Input: part model. Units: mm. Frame: model coordinates. A direction names the side the tool comes from. Give positions to 0.01 mm unless a question says otherwise; leave off trailing zeros. Loops run counter-clockwise (first coordinate to the right, second up) from the corner with the lowest first, then second, coordinate; pieces in that order, holes last.
from build123d import *

# Parameters (mm, degrees)
SKETCH1_R           = 5.375
SKETCH1_R_2         = 3.375
BOSS_EXTRUDE1_DEPTH = 12
FILLET1_R           = 10
FILLET1_2_R         = 6
CHAMFER1_SIZE       = 1


with BuildPart() as part:
    # Sketch1 → Boss-Extrude1 (new body)
    with BuildSketch(Plane.XY):
        Circle(SKETCH1_R)
        Circle(SKETCH1_R_2, mode=Mode.SUBTRACT)
        with BuildLine():
            Line((13.516056888, 82), (2.713546265, 82))
            Line((2.713546265, 82), (-5.348872315, 0.529329726))
            ThreePointArc((-5.348872315, 0.529329726), (0.264987082, 5.368464105), (5.375, 0))
            ThreePointArc((5.375, 0), (5.368464105, -0.264987082), (5.348872315, -0.529329726))
            Line((5.348872315, -0.529329726), (13.516056888, 82))
        make_face()
        Polygon((14.307744846, 90), (3.505234224, 90), (2.713546265, 82), (13.516056888, 82), align=None)
        Polygon((46.473934517, 90), (14.307744846, 90), (13.516056888, 82), (46.473934517, 82), align=None)
    extrude(amount=BOSS_EXTRUDE1_DEPTH)

    # Fillet1
    fillet1_edges = [part.edges().sort_by_distance(p)[0] for p in [
        (3.505234224, 90, 6),
    ]]
    fillet(fillet1_edges, radius=FILLET1_R)

    # Fillet1 2
    fillet1_2_edges = [part.edges().sort_by_distance(p)[0] for p in [
        (13.516056888, 82, 6),
    ]]
    fillet(fillet1_2_edges, radius=FILLET1_2_R)

    # Chamfer1
    chamfer1_edges = [part.edges().sort_by_distance(p)[0] for p in [
        (-0.529329726, -5.348872315, 12),
        (-0.529329726, -5.348872315, 0),
        (32.712766845, 82, 12),
        (9.164818638, 38.030774984, 0),
        (9.164818638, 38.030774984, 12),
        (-1.367895651, 40.757064607, 0),
        (-1.367895651, 40.757064607, 12),
        (29.519202941, 90, 0),
        (5.850604928, 87.411072625, 0),
        (29.519202941, 90, 12),
        (5.850604928, 87.411072625, 12),
        (14.92327931, 80.446643575, 0),
        (14.92327931, 80.446643575, 12),
        (32.712766845, 82, 0),
    ]]
    chamfer(chamfer1_edges, length=CHAMFER1_SIZE)


solid = part.part
(1) Mould query, pull axis Z, two halves, no side actions, for faces 1 (the cylindrical face through (-0.647, -5.336, 5.93)), 2 (the flat face through (8.607, 37.541, 11.507)), 3 (the flat face through (-0.822, 41.272, 0.507)). Classes: +Z half, -Z half, draft (parallel to the pull), parting line (faces both ways), or undercut.
Values follow:
face 1: draft
face 2: +Z half
face 3: -Z half
(2) Cut plane A-A (x = 29.5). Return the cut outline in (y, z).
Values follow:
outline: (82, 1) - (83, 0) - (89, 0) - (90, 1) - (90, 11) - (89, 12) - (83, 12) - (82, 11) - close
(3) Reachability of faces 4 (the flat face through (33, 82, 6)), 5 (the conical face through (14.76, 80.53, 11.17)) from +Z, -Z, +X, -X, +Y, -Y: full face, straight path, thin tool, end or side. Return the list, or none.
Values follow:
face 4: +Z, -Z, +X, -Y
face 5: +Z, +X, -Y
(4) Cut plane B-B (y = 2). Return the cut outline in (x, z), and give its area (3 significant figures).
Values follow:
outline: (-5.2, 1) - (-4.2, 0) - (-2.72, 0) - (-2.72, 12) - (-4.2, 12) - (-5.2, 11) - close; (2.72, 0) - (4.59, 0) - (5.6, 1) - (5.6, 11) - (4.59, 12) - (2.72, 12) - close
area: 62.4 mm2
(5) Pin query (flat end, axial travel): pin 1 Ø1 at (y, z) = (17, 7) entering from -X. Return the tip coordinate at first contact, or that it passes through.
Values follow:
pin 1: stops at x = -3.77
(6) Cut plane C-C (x = 0). Return the cut outline in (y, z) (3 decimals).
Values follow:
outline: (-5.375, 1) - (-4.375, 0) - (-3.375, 0) - (-3.375, 12) - (-4.375, 12) - (-5.375, 11) - close; (3.375, 0) - (44.425, 0) - (54.58, 1) - (54.58, 11) - (44.425, 12) - (3.375, 12) - close
(7) Ray query, probe 1 along Y at (x, z) = (32, 4.25); probe 2 along X at (y, z) = (1.5, 0.5); probe 3 along X at (y, z) = (33, 8.5). Return the intervals inside material, ascending.
Values follow:
probe 1: y = 82 to 90
probe 2: x = -4.75 to -3.02, 3.02 to 5.05
probe 3: x = -2.14 to 8.67
